For this review, use the dimensioned drawing (mm, ordinates from the lowest corner) and the shaded views. A direction names the side the tool comes from. Give positions to 0.01 mm unless a question says otherwise; leave off trailing zeros. Order: outer loops, then holes, each group sorted by start corner. A loop starts at its lowest first (then second) coordinate and runs counter-clockwise, first axis right, second up.
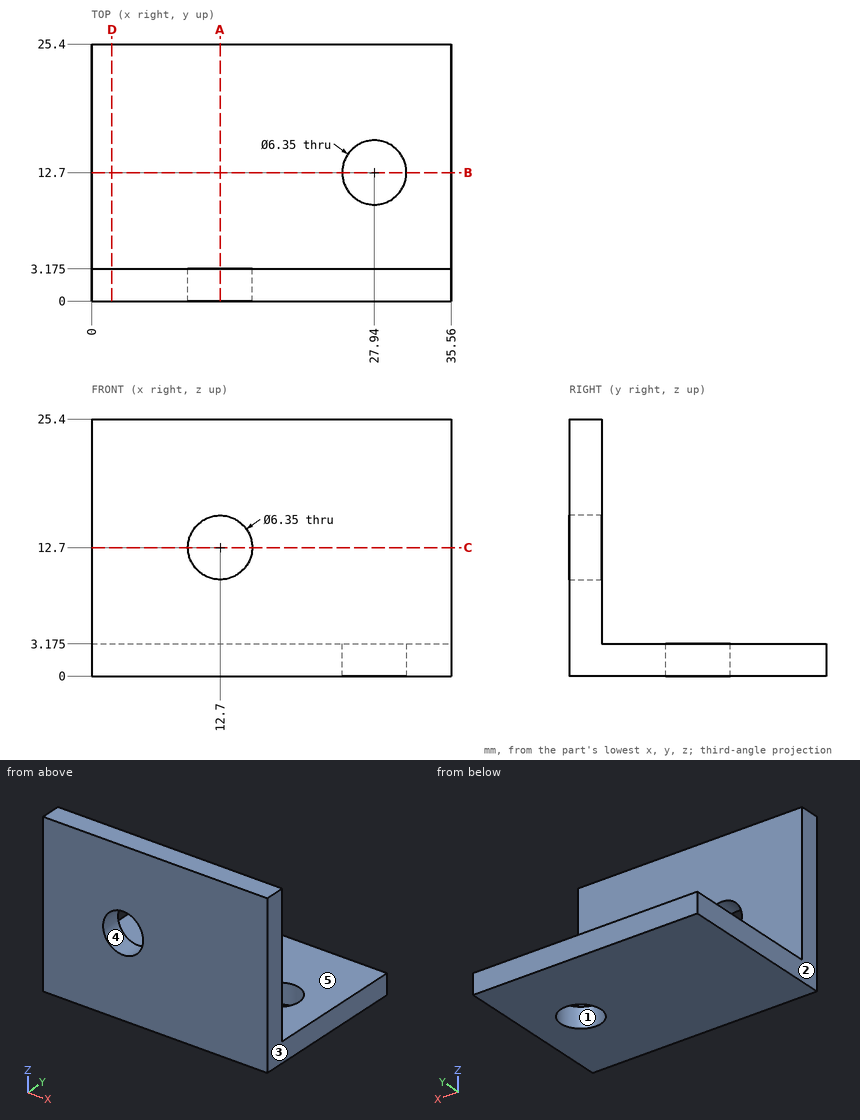
1. Take a section at A-A (x = 12.7). State the section outline as (y, z) points (3 decimals), then the cut area to 3 significant figures.
Recorded:
outline: (0, 0) - (25.4, 0) - (25.4, 3.175) - (3.175, 3.175) - (3.175, 9.525) - (0, 9.525) - close; (0, 15.875) - (3.175, 15.875) - (3.175, 25.4) - (0, 25.4) - close
area: 131 mm2
2. Draft analysis for pull direction X (two halves, no side actions). For the marked faces 1, 2 and 3, state which applies: pulls with the +X half, pulls with the -X half, needs draft (parallel to the pull), parting line crosses it, or undercut.
Recorded:
face 1: undercut
face 2: pulls with the -X half
face 3: pulls with the +X half
3. Machinability: for the marked faces 4 and 5, which of the approach directions +Z, -Z, +X, -X, +Y, -Y give a long, thin tool a straight path to every point of the face, cutting with its end or side? Answer none if there is none.
Recorded:
face 4: +Y, -Y
face 5: +Z, +X, -X, +Y
4. Take a section at C-C (z = 12.7). State the section outline as (x, y) points (3 decimals).
Recorded:
outline: (0, 0) - (9.525, 0) - (9.525, 3.175) - (0, 3.175) - close; (15.875, 0) - (35.56, 0) - (35.56, 3.175) - (15.875, 3.175) - close
5. For pin 1 (4 mm diameter, centred on x = 20.5, z = 20, fed in from +Y) (3 decimals); pin 2 (10 mm diameter, centred on x = 27.94, y = 12.7, fed in from +Z) (3 decimals), all flat-tipped, find the tip position at first contact; note any pin that passes through.
Recorded:
pin 1: stops at y = 3.175
pin 2: stops at z = 3.175
6. Take a section at D-D (x = 2). State the section outline as (y, z) points (3 decimals), then the cut area to 3 significant figures.
Recorded:
outline: (0, 0) - (25.4, 0) - (25.4, 3.175) - (3.175, 3.175) - (3.175, 25.4) - (0, 25.4) - close
area: 151 mm2
7. Take a section at B-B (y = 12.7). State the section outline as (x, z) points (3 decimals).
Recorded:
outline: (0, 0) - (24.765, 0) - (24.765, 3.175) - (0, 3.175) - close; (31.115, 0) - (35.56, 0) - (35.56, 3.175) - (31.115, 3.175) - close
8. For line 1 along Y through (x, z) = (27.94, 0.8) (3 decimals); line 2 along X through (y, z) = (1.4, 12.7) (3 decimals); line 3 along Z through (x, y) = (32, 23.25) (3 decimals), list the stretches that pass through material, from the lowest coordinate up.
Recorded:
line 1: y = 0 to 9.525, 15.875 to 25.4
line 2: x = 0 to 9.525, 15.875 to 35.56
line 3: z = 0 to 3.175
